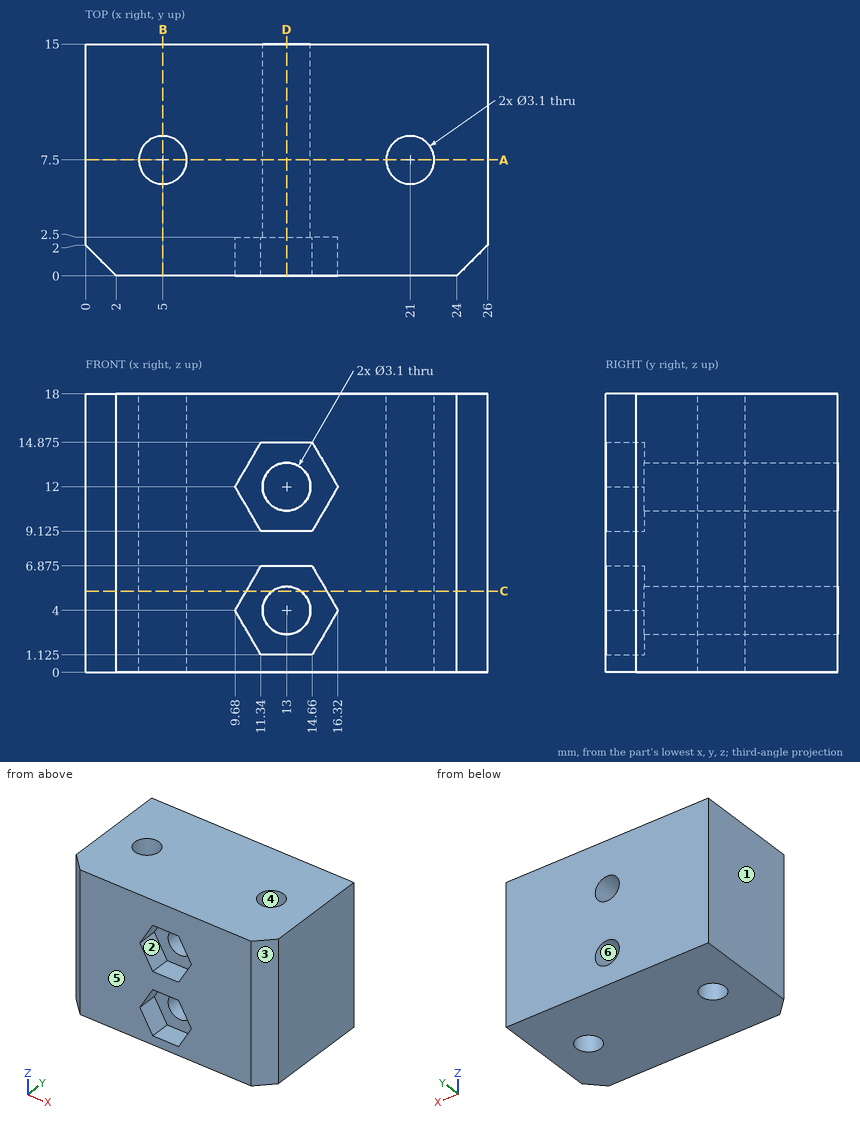
Geometry check sheet. Reference: drawing and pictorial views, mm from the part's lowest x, y, z. A direction names the side the tool comes from. Coordinates: 2 decimals unless noted, no trailing zeros. Order: outer loops, then holes, each group sorted by start corner. A loop starts at its lowest first (then second) coordinate and runs counter-clockwise, first axis right, second up. Notation, with made-up numbers: M 58.5,57.25 L 96.5,57.25 A28 cw 96.5,82.25 Z; hole C 63,7.25 d1. An arc over 180 degrees is marked long. Return JSON: item names as keys, results as strings.
1) Access from +Z, -Z, +X, -X, +Y, -Y to the whole of each face (thin tool, end or side, straight path). Record for the marked faces 1 and 2.
Answer list:
{"face 1": "+Z, -Z, -X, +Y, -Y", "face 2": "-Y"}
2) Cross-section at B-B, the plane x = 5. Record the boundary of the cut face in (y, z), and give its area (3 significant figures).
Answer list:
{"outline": "M 0,0 L 5.95,0 L 5.95,18 L 0,18 Z; M 9.05,0 L 15,0 L 15,18 L 9.05,18 Z", "area": "214 mm2"}
3) Thickness scan on L1, parallel to X at y = 5, z = 4; L2, parallel to Z at x = 13, y = 9; L3, parallel to X at y = 7.75, z = 12. Record the ranges inside material, lowest first. Write a range as [from, to].
Answer list:
{"L1": "[0, 11.45], [14.55, 26]", "L2": "[0, 2.45], [5.55, 10.45], [13.55, 18]", "L3": "[0, 3.47], [6.53, 11.45], [14.55, 19.47], [22.53, 26]"}
4) Cross-section at A-A, the plane y = 7.5. Record the boundary of the cut face in (x, z), and give its area (3 significant figures).
Answer list:
{"outline": "M 0,0 L 3.45,0 L 3.45,18 L 0,18 Z; M 6.55,0 L 19.45,0 L 19.45,18 L 6.55,18 Z; M 22.55,0 L 26,0 L 26,18 L 22.55,18 Z; hole C 13,4 d3.1; hole C 13,12 d3.1", "area": "341 mm2"}
5) Gauge pin test, flat ends, axial feed: pin 1 (2.5 mm diameter, centred on x = 13, z = 4, fed in from +Y); pin 2 (4.5 mm diameter, centred on x = 13.5, z = 4, fed in from -Y). Record the tip position at first contact, or that the pin passes through.
Answer list:
{"pin 1": "through", "pin 2": "y = 2.5"}
6) Cross-section at D-D, the plane x = 13. Record the boundary of the cut face in (y, z) (3 decimals).
Answer list:
{"outline": "M 0,0 L 15,0 L 15,2.45 L 2.5,2.45 L 2.5,1.125 L 0,1.125 Z; M 0,6.875 L 2.5,6.875 L 2.5,5.55 L 15,5.55 L 15,10.45 L 2.5,10.45 L 2.5,9.125 L 0,9.125 Z; M 0,14.875 L 2.5,14.875 L 2.5,13.55 L 15,13.55 L 15,18 L 0,18 Z"}
7) Release check for a two-part mould opening along X. For the marked faces 3, 4, 5 and 6 record: +X half, -X half, draft (parallel to the pull), parting line (faces both ways), or undercut.
Answer list:
{"face 3": "+X half", "face 4": "undercut", "face 5": "draft", "face 6": "undercut"}
8) Cross-section at C-C, the plane z = 5.25. Record the boundary of the cut face in (x, y), and give its area (3 significant figures).
Answer list:
{"outline": "M 0,2 L 2,0 L 10.4,0 L 10.4,2.5 L 12.08,2.5 L 12.08,15 L 0,15 Z; M 13.92,2.5 L 15.6,2.5 L 15.6,0 L 24,0 L 26,2 L 26,15 L 13.92,15 Z; hole C 5,7.5 d3.1; hole C 21,7.5 d3.1", "area": "335 mm2"}
